from build123d import *

# Parameters (mm, degrees)
F0_R     = 12.5
F1_DEPTH = 17.5


with BuildPart() as f1:
    # F0 (on Front) → F1 (new body)
    with BuildSketch(Plane.XZ):
        with BuildLine():
            Line((-45.037766, 9.175865), (-5.037766, 9.175865))
            Line((-5.037766, 9.175865), (-5.037766, 12.45487))
            Line((-5.037766, 12.45487), (-0.037766, 12.45487))
            Line((-0.037766, 12.45487), (-0.037766, 27.45487))
            Line((-0.037766, 27.45487), (-5.037766, 27.45487))
            Line((-5.037766, 27.45487), (-5.037766, 42.45487))
            ThreePointArc((-5.037766, 42.45487), (-25.037766, 62.45487), (-45.037766, 42.45487))
            Line((-45.037766, 42.45487), (-45.037766, 27.45487))
            Line((-45.037766, 27.45487), (-50.037766, 27.45487))
            Line((-50.037766, 27.45487), (-50.037766, 12.45487))
            Line((-50.037766, 12.45487), (-45.037766, 12.45487))
            Line((-45.037766, 12.45487), (-45.037766, 9.175865))
        make_face()
        with Locations((-25.037766, 42.45487)):
            Circle(F0_R, mode=Mode.SUBTRACT)
    extrude(amount=F1_DEPTH)


solid = f1.part
The model under review builds one solid part; all positions refer to its coordinate system, in mm. A direction names the side the tool comes from. Give positions to 0.01 mm unless a question says otherwise; leave off trailing zeros. Order: outer loops, then holes, each group sorted by start corner. A loop starts at its lowest first (then second) coordinate and runs counter-clockwise, first axis right, second up. Notation, with made-up numbers: M -6,65.25 L 7,65.25 A20 ccw 7,93.25 Z; hole C 2,21.5 d10. An arc over 180 degrees is marked long. One line per question, with ' | ' between items. Start each with the question number.
1) Consider section B-B, the plane z = 34.5. Give the boundary of the cut face in (x, y), then the cut area to 3 significant figures.
2) Clearance check with flat-ended pins moving along their axes: P1, Ø1.5, axis at x = -3.5, y = -11, coming from the +Z side; P2, Ø1.5, axis at x = -3.5, y = -10, coming from the -Z side; P3, Ø7.5, axis at y = -10.5, z = 31.5, coming from the -X side. State where each tip first meets the part, or that it passes through.
3) Consider section D-D, the plane x = -11.5. Give the boundary of the cut face in (y, z).
4) For faces 1 (the face through (-3, -9, 27.455)), 2 (the face through (-5.038, -9, 11)), 3 (the face through (-31, 0, 30)), 4 (the face through (-45.038, -9, 35)), 5 (the face through (-48, -9, 12.455)), list the 3-axis set-ups (+Z, -Z, +X, -X, +Y, -Y) from which the entire face can be reached by the end or side of a thin tool; tool diameter is ignored.
5) Wall thickness on L1, parallel to Z at x = -25, y = -9.5; L2, parallel to Z at x = -16, y = -2.5; L3, parallel to X at y = -12.25, z = 39: over which ranges is each line inside the solid? List them lowest first. Write a range as from..to.
6) Consider section C-C, the plane y = -7.25. Give the boundary of the cut face in (x, z), then the cut area to 3 significant figures.
7) Consider section A-A, the plane x = -22.5. Give the boundary of the cut face in (y, z).
Found:
1) outline: M -45.04,-17.5 L -34.68,-17.5 L -34.68,0 L -45.04,0 Z; M -15.4,-17.5 L -5.04,-17.5 L -5.04,0 L -15.4,0 Z | area: 363 mm²
2) P1: stops at z = 27.45 | P2: stops at z = 12.45 | P3: stops at x = -45.04
3) outline: M -17.5,9.18 L 0,9.18 L 0,57.18 L -17.5,57.18 Z
4) face 1: +Z, +X, +Y, -Y | face 2: -Z, +X, +Y, -Y | face 3: +Z, -Z, +X, -X, +Y | face 4: +Z, -X, +Y, -Y | face 5: -Z, -X, +Y, -Y
5) L1: z = 9.18..29.95, 54.95..62.45 | L2: z = 9.18..33.82, 51.09..60.3 | L3: x = -45.04..-37.05, -13.02..-5.04
6) outline: M -50.04,12.45 L -45.04,12.45 L -45.04,9.18 L -5.04,9.18 L -5.04,12.45 L -0.04,12.45 L -0.04,27.45 L -5.04,27.45 L -5.04,42.45 A20 ccw -45.04,42.45 L -45.04,27.45 L -50.04,27.45 Z; hole C -25.04,42.45 d25 | area: 1,620 mm²
7) outline: M -17.5,9.18 L 0,9.18 L 0,30.22 L -17.5,30.22 Z; M -17.5,54.69 L 0,54.69 L 0,62.29 L -17.5,62.29 Z
